Geometry: final body of the model. Coordinates: model frame, mm. Round coordinates to 2 decimals unless told otherwise and drop trailing zeros. Order: outer loops, then holes, each group sorted by start corner. A loop starts at its lowest first (then second) coordinate and runs counter-clockwise, first axis right, second up. Notation, with made-up numbers: M -5.5,-33.75 L 16.5,-33.75 A23 cw 16.5,2.25 Z; hole C 59,-19 d3. An arc over 180 degrees is marked long. Return JSON: item names as keys, results as strings. Group by question number.
Q1. Ray query, probe 1 along Y at (x, z) = (3, 1.95); probe 2 along Y at (x, z) = (3, 4.65); probe 3 along X at (y, z) = (35, 3). Return the intervals inside material, ascending.
Q2. Contact query for flat-ended pins moving along their axis: pin 1 (2 mm diameter, centred on y = 62.5, z = 2.5, fed in from -X); pin 2 (3 mm diameter, centred on x = 3, z = 2.5, fed in from +Y); pin 3 (2 mm diameter, centred on x = -123, z = 0.5, fed in from +Y); pin 4 (2.5 mm diameter, centred on x = 3, y = 48.3, fed in from +Z). Output: stop coordinate, or through.
Q3. Cut plane B-B on x = -118. Output: boundary loops of the cut face in (y, z), and give its area (3 significant figures).
Q4. Cut plane A-A on z = 5. Output: boundary loops of the cut face in (x, y) (3 decimals).
Q5. Cut plane C-C on y = 80.5. Output: boundary loops of the cut face in (x, z).
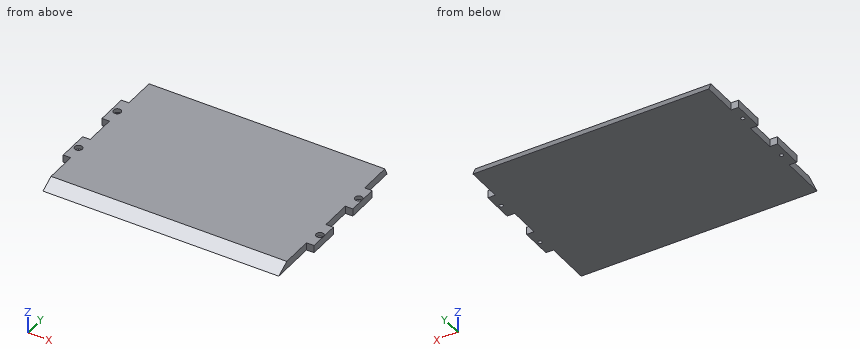
```python
from build123d import *

# Parameters (mm, degrees)
ESQUISSE1_W                  = 188
ESQUISSE1_H                  = 139.6
BOSS_EXTRU_1_DEPTH           = 6
ENL_V_START                  = -189
ENL_V_MAT_EXTRU_3_DEPTH      = 190
ENL_V_MAT_EXTRU_4_DEPTH      = 235.239535519
ENL_V_MAT_EXTRU_4_DEPTH_BACK = 235.239535519
ESQUISSE7_W                  = 6
ESQUISSE7_H                  = 25
BOSS_EXTRU_3_DEPTH           = 6
ESQUISSE9_W                  = 6
ESQUISSE9_H                  = 25
BOSS_EXTRU_4_DEPTH           = 6
ESQUISSE11_R                 = 2.995
ENL_V_MAT_EXTRU_7_DEPTH      = 3
ESQUISSE12_R                 = 1.5
ENL_V_MAT_EXTRU_8_DEPTH      = 13


with BuildPart() as part:
    # Esquisse1 → Boss.-Extru.1 (new body)
    with BuildSketch(Plane.XY):
        with Locations((-94, 69.8)):
            Rectangle(ESQUISSE1_W, ESQUISSE1_H)
    extrude(amount=BOSS_EXTRU_1_DEPTH)

    # Enlèv. mat.-Extru.3: read off the stored shape, not the designer's step
    # Enlèv. mat.-Extru.3 outline → Enlèv. mat.-Extru.3 (cut)
    with BuildSketch(Plane(origin=(0, 0, 0), x_dir=(0, 0, -1), z_dir=(1, 0, 0)).offset(ENL_V_START)):
        Polygon((-6, 139.6), (-6, 136.802154051), (0, 139.6), align=None)
    extrude(amount=ENL_V_MAT_EXTRU_3_DEPTH, mode=Mode.SUBTRACT)

    # Esquisse4 → Enlèv. mat.-Extru.4 (cut, two sides: drawn at the far end of the back side and taken through both)
    with BuildSketch(Plane(origin=(0, 0, 0), x_dir=(0, 0, -1), z_dir=(1, 0, 0)).offset(-ENL_V_MAT_EXTRU_4_DEPTH_BACK)):
        Polygon((144.728880336, -250.677774065), (0, 0), (-6, 10.392304845), (-150.728880336, 261.07007891), (-652.084428466, -28.387681762), (-356.626667793, -540.135534737), align=None)
    extrude(amount=ENL_V_MAT_EXTRU_4_DEPTH + ENL_V_MAT_EXTRU_4_DEPTH_BACK, mode=Mode.SUBTRACT)

    # Esquisse7 → Boss.-Extru.3 (add)
    with BuildSketch(Plane(origin=(0, 0, 0), x_dir=(0, 0, -1), z_dir=(1, 0, 0))):
        with Locations((-3, 98.302154051)):
            Rectangle(ESQUISSE7_W, ESQUISSE7_H)
        with Locations((-3, 48.302154051)):
            Rectangle(ESQUISSE7_W, ESQUISSE7_H)
    extrude(amount=BOSS_EXTRU_3_DEPTH)

    # Esquisse9 → Boss.-Extru.4 (add)
    with BuildSketch(Plane.ZY.offset(188)):
        with Locations((3, 48.302154051)):
            Rectangle(ESQUISSE9_W, ESQUISSE9_H)
        with Locations((3, 98.302154051)):
            Rectangle(ESQUISSE9_W, ESQUISSE9_H)
    extrude(amount=BOSS_EXTRU_4_DEPTH)

    # Esquisse11 → Enlèv. mat.-Extru.7 (cut)
    with BuildSketch(Plane.XY.offset(6)):
        with Locations((3, 48.302154051)):
            Circle(ESQUISSE11_R)
        with Locations((3, 98.302154051)):
            Circle(ESQUISSE11_R)
        with Locations((-189.537877077, 48.302154051)):
            Circle(ESQUISSE11_R)
        with Locations((-189.537877077, 98.302154051)):
            Circle(ESQUISSE11_R)
    extrude(amount=-ENL_V_MAT_EXTRU_7_DEPTH, mode=Mode.SUBTRACT)

    # Esquisse12 → Enlèv. mat.-Extru.8 (cut)
    with BuildSketch(Plane.XY.offset(6)):
        with Locations((3, 98.302154051)):
            Circle(ESQUISSE12_R)
        with Locations((3, 48.302154051)):
            Circle(ESQUISSE12_R)
        with Locations((-189.537877077, 48.302154051)):
            Circle(ESQUISSE12_R)
        with Locations((-189.537877077, 98.302154051)):
            Circle(ESQUISSE12_R)
    extrude(amount=-ENL_V_MAT_EXTRU_8_DEPTH, mode=Mode.SUBTRACT)


solid = part.part
```
Result sheet:
{
 "1": {"probe 1": "y = 35.8 to 46.8, 49.8 to 60.8, 85.8 to 96.8, 99.8 to 110.8", "probe 2": "y = 35.8 to 45.31, 51.3 to 60.8, 85.8 to 95.31, 101.3 to 110.8", "probe 3": "x = -188 to 0"},
 "2": {"pin 1": "stops at x = -188", "pin 2": "stops at y = 110.8", "pin 3": "stops at y = 139.6", "pin 4": "passes through"},
 "3": {"outline": "M 0,0 L 139.6,0 L 136.8,6 L 10.39,6 Z", "area": "798 mm²"},
 "4": {"outline": "M -194,35.802 L -188,35.802 L -188,8.66 L 0,8.66 L 0,35.802 L 6,35.802 L 6,60.802 L 0,60.802 L 0,85.802 L 6,85.802 L 6,110.802 L 0,110.802 L 0,137.268 L -188,137.268 L -188,110.802 L -194,110.802 L -194,85.802 L -188,85.802 L -188,60.802 L -194,60.802 Z; hole C -189.538,48.302 d5.99; hole C -189.538,98.302 d5.99; hole C 3,48.302 d5.99; hole C 3,98.302 d5.99"},
 "5": {"outline": "M -188,0 L 0,0 L 0,6 L -188,6 Z"}
}
